Here's how the part is built. I have some questions about the finished solid (model axes, mm). A direction names the side the tool comes from. Coordinates: 2 decimals unless noted, no trailing zeros. Loops run counter-clockwise (first coordinate to the right, second up) from the corner with the lowest first, then second, coordinate; pieces in that order, holes last. Notation, with made-up numbers: (67, 19) -> (114, 19) arc R28 ccw to (114, 58) -> close; hole circle Ø5 at (-7.5, -39). An arc over 180 degrees is marked (long way). Answer as a JSON object with one key per item and string values. Group by question number.
1) I need wall thicknesses on probe 1 along Z at (x, y) = (0, 4.25) (3 decimals); probe 2 along Z at (x, y) = (0, -0.2); probe 3 along X at (y, z) = (1.75, -3.75). Which ranges of each line are inside material? Lowest first, please. Write a range as [from, to].
2) I want a section at C-C (y = 3). Write out the boundary of the cut face in (x, z) (3 decimals), then the cut area to 3 significant figures.
3) I want a section at A-A (x = 0). Write out the boundary of the cut face in (y, z) (3 decimals), then the cut area to 3 significant figures.
4) I'm going to push flat-ended pins straight in: pin 1 (1.5 mm diameter, centred on x = -5.5, y = 0.5, fed in from -Z); pin 2 (1 mm diameter, centred on y = 2, z = -11, fed in from -X); pin 3 (1 mm diameter, centred on x = 5.5, z = 10, fed in from -Y). Where does each tip first touch, or does it pass through?
5) I want a section at B-B (z = 0). Write out the boundary of the cut face in (x, y) (3 decimals), then the cut area to 3 significant figures.
6) If we mould it in two halves opening along Z, with no side actions, what happens to faces 3 (the flat face through (5.1, 7.2, 12.4)), 4 (the cylindrical face through (7.91, 3.277, 10.316)), 5 (the cylindrical face through (7.32, 3.92, 9.54))? For each: +Z half, -Z half, draft (parallel to the pull), parting line (faces both ways), or undercut.
7) Which directions (+Z, -Z, +X, -X, +Y, -Y) give clear straight access to the entire face, cutting with the end or side of a thin tool? Please do faces 1 (the flat face through (9, 8.2, -9)), 2 (the flat face through (-5, 0, 10)).
```python
from build123d import *


with BuildPart() as part:
    # Sketch1 → Revolve1 (revolve)
    with BuildSketch(Plane(origin=(0, 0, 0), x_dir=(0, 0, -1), z_dir=(1, 0, 0))):
        with BuildLine():
            Line((11, 0), (11, -0.5))
            Line((11, -0.5), (11.5, -1))
            Line((11.5, -1), (12.5, -1))
            Line((12.5, -1), (13, -0.5))
            Line((13, -0.5), (13, 6.95))
            ThreePointArc((13, 6.95), (13.073223305, 7.126776695), (13.25, 7.2))
            Line((13.25, 7.2), (14, 7.2))
            Line((14, 7.2), (14, 7.7))
            Line((14, 7.7), (13.5, 8.2))
            Line((13.5, 8.2), (12.525, 8.2))
            Line((12.525, 8.2), (12.025, 7.7))
            Line((12.025, 7.7), (12.025, 0.25))
            ThreePointArc((12.025, 0.25), (11.951776695, 0.073223305), (11.775, 0))
            Line((11.775, 0), (11, 0))
        make_face()
    revolve(axis=Axis((0, 0, 0), (0, 1, 0)))


solid = part.part
```
Determined:
{
 "1": {"probe 1": "[-13, -12.025], [12.025, 13]", "probe 2": "[-13, -11], [11, 13]", "probe 3": "[-12.45, -11.43], [11.43, 12.45]"},
 "2": {"outline": "circle Ø26 at (0, 0); hole circle Ø24.05 at (0, 0)", "area": "76.7 mm^2"},
 "3": {"outline": "(-1, -12.5) -> (-0.5, -13) -> (6.95, -13) arc R0.25 cw to (7.2, -13.25) -> (7.2, -14) -> (7.7, -14) -> (8.2, -13.5) -> (8.2, -12.525) -> (7.7, -12.025) -> (0.25, -12.025) arc R0.25 cw to (0, -11.775) -> (0, -11) -> (-0.5, -11) -> (-1, -11.5) -> close; (-1, 11.5) -> (-0.5, 11) -> (0, 11) -> (0, 11.775) arc R0.25 cw to (0.25, 12.025) -> (7.7, 12.025) -> (8.2, 12.525) -> (8.2, 13.5) -> (7.7, 14) -> (7.2, 14) -> (7.2, 13.25) arc R0.25 cw to (6.95, 13) -> (-0.5, 13) -> (-1, 12.5) -> close", "area": "21.0 mm^2"},
 "4": {"pin 1": "z = -12.1", "pin 2": "x = -7.66", "pin 3": "y = -1"},
 "5": {"outline": "(-14, 7.2) -> (-13.25, 7.2) arc R0.25 cw to (-13, 6.95) -> (-13, -0.5) -> (-12.5, -1) -> (-11.5, -1) -> (-11, -0.5) -> (-11, 0) -> (-11.775, 0) arc R0.25 cw to (-12.025, 0.25) -> (-12.025, 7.7) -> (-12.525, 8.2) -> (-13.5, 8.2) -> (-14, 7.7) -> close; (11, -0.5) -> (11.5, -1) -> (12.5, -1) -> (13, -0.5) -> (13, 6.95) arc R0.25 cw to (13.25, 7.2) -> (14, 7.2) -> (14, 7.7) -> (13.5, 8.2) -> (12.525, 8.2) -> (12.025, 7.7) -> (12.025, 0.25) arc R0.25 cw to (11.775, 0) -> (11, 0) -> close", "area": "21.0 mm^2"},
 "6": {"face 3": "draft", "face 4": "parting line", "face 5": "undercut"},
 "7": {"face 1": "+Z, -Z, +X, -X, +Y", "face 2": "+Y"}
}
